Here's how the part is built. I have some questions about the finished solid (model axes, mm). Face numbers are marked on the shaded views. Coordinates: 2 decimals unless noted, no trailing zeros. Order: outer loops, then holes, each group sorted by start corner. A loop starts at its lowest first (then second) coordinate and runs counter-clockwise, first axis right, second up. Notation, with made-up numbers: (29, 19) - (58, 19) arc R15 cw to (58, 27) - close; hole circle Ø10 at (24.5, 38). An arc over 180 degrees is marked (long way). Answer in a Markdown table with one row per item. Add a question column.
Item 1: I want a section at B-B (x = 0). Please give me the cut outline in (y, z).
Item 2: I want a section at C-C (y = 1.85). Please give me the cut outline in (x, z).
Item 3: I want a section at A-A (z = 0). Please give me the cut outline in (x, y), plus the area to 3 significant figures.
Item 4: I want a section at D-D (z = -2.5). Please give me the cut outline in (x, y), plus the area to 3 significant figures.
Item 5: Thinking about a two-plate mould opening in X: for the marked faces 1, 2 and 3, which applies, +X half, -X half, draft (parallel to the pull), parting line (faces both ways), or undercut?
Item 6: If I drill on line 1 along Z through (x, y) = (0, 2.1); line 2 along Y through (x, z) = (0.25, 3.75), over which ranges is the centre line in solid material (lowest first)? Write a range as from..to.
Item 7: Will this pin go through, and if not, where does the flat tip stop? pin 1 Ø4 at (x, z) = (2, 4.5) entering from +Y.
Autodesk Inventor part; units mm, degrees
ref_plane "YZ Plane" through (0, 0, 0) normal (1, 0, 0) x (0, 1, 0)
ref_plane "XZ Plane" through (0, 0, 0) normal (0, 1, 0) x (-1, 0, 0)
ref_plane "XY Plane" through (0, 0, 0) normal (0, 0, 1) x (1, 0, 0)
sketch "スケッチ1" plane through (0, 0, 0) normal (0, 1, 0) x (-1, 0, 0)
  circle A0 centre (0, 0) radius 6
  dimension "d0" = 12
extrude "押し出し1" add sketch "スケッチ1" along normal blind 1
sketch "スケッチ2" plane through (0, 1, 0) normal (0, 1, 0) x (1, 0, 0)
  circle A0 centre (0, 0) radius 3
  dimension "d3" = 6
extrude "押し出し2" add sketch "スケッチ2" along normal blind 3
sketch "スケッチ3" plane through (0, 4, 0) normal (0, 1, 0) x (1, 0, 0)
  circle A0 centre (0, 0) radius 1.9
  dimension "d6" = 3.8
extrude "押し出し3" cut sketch "スケッチ3" against normal through all
properties part number "ベルト_bush"
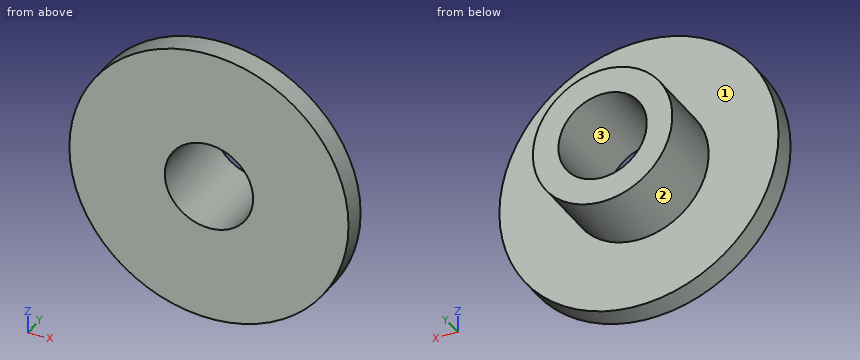
Values follow:
| question | item | result |
|---|---|---|
| 1 | outline | (0, -6) - (1, -6) - (1, -3) - (4, -3) - (4, -1.9) - (0, -1.9) - close; (0, 1.9) - (4, 1.9) - (4, 3) - (1, 3) - (1, 6) - (0, 6) - close |
| 2 | outline | circle Ø6 at (0, 0); hole circle Ø3.8 at (0, 0) |
| 3 | outline | (-6, 0) - (-1.9, 0) - (-1.9, 4) - (-3, 4) - (-3, 1) - (-6, 1) - close; (1.9, 0) - (6, 0) - (6, 1) - (3, 1) - (3, 4) - (1.9, 4) - close |
| 3 | area | 14.8 mm^2 |
| 4 | outline | (-5.45, 0) - (5.45, 0) - (5.45, 1) - (1.66, 1) - (1.66, 4) - (-1.66, 4) - (-1.66, 1) - (-5.45, 1) - close |
| 4 | area | 20.9 mm^2 |
| 5 | face 1 | draft |
| 5 | face 2 | parting line |
| 5 | face 3 | undercut |
| 6 | line 1 | z = -3..-1.9, 1.9..3 |
| 6 | line 2 | y = 0..1 |
| 7 | pin 1 | stops at y = 4 |
